Read the model definition and answer for the solid it produces. Units are mm, in the model's axes. Face numbers are marked on the shaded views. A direction names the side the tool comes from. Coordinates: 2 decimals unless noted, no trailing zeros. Order: outer loops, then holes, each group sorted by start corner. A loop starts at its lowest first (then second) coordinate and runs counter-clockwise, first axis right, second up. Notation, with made-up numbers: (79.5, 17) -> (121.5, 17) arc R15 ccw to (121.5, 30) -> close; hole circle Ø2 at (4, -16). An arc over 180 degrees is marked (long way). Answer in a Markdown table with one row per item.
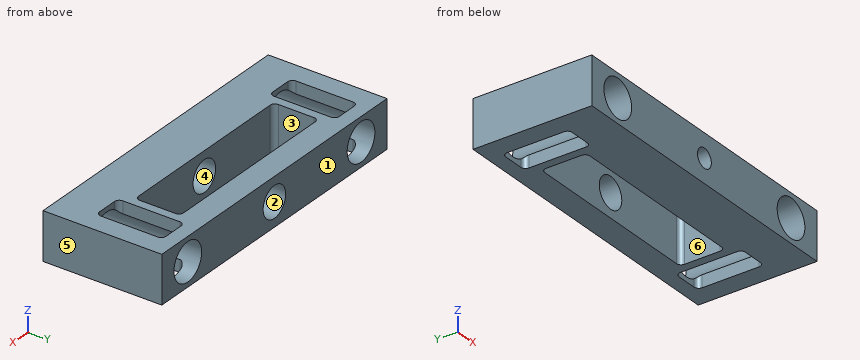
from build123d import *

# Parameters (mm, degrees)
SKETCH1_W                = 130
SKETCH1_H                = 50
BOSS_EXTRUDE1_DEPTH      = 10
BOSS_EXTRUDE1_DEPTH_BACK = 10
SKETCH2_R                = 8
CUT_EXTRUDE1_DEPTH       = 1
CUT_EXTRUDE1_DEPTH_BACK  = 51
CUT_EXTRUDE2_DEPTH       = 23
SKETCH5_R                = 4
CUT_EXTRUDE3_DEPTH       = 1.0000001
CUT_EXTRUDE3_DEPTH_BACK  = 51.0000001
SKETCH6_R                = 6.5
CUT_EXTRUDE4_DEPTH       = 37.5


with BuildPart() as part:
    # Sketch1 → Boss-Extrude1 (new body, two sides)
    with BuildSketch(Plane.XY) as boss_extrude1_sk:
        with Locations((0, -5)):
            Rectangle(SKETCH1_W, SKETCH1_H)
        with BuildLine():
            Line((38, 9.5), (-38, 9.5))
            ThreePointArc((-38, 9.5), (-39.414213562, 8.914213562), (-40, 7.5))
            Line((-40, 7.5), (-40, -7.5))
            ThreePointArc((-40, -7.5), (-39.414213562, -8.914213562), (-38, -9.5))
            Line((-38, -9.5), (38, -9.5))
            ThreePointArc((38, -9.5), (39.414213562, -8.914213562), (40, -7.5))
            Line((40, -7.5), (40, 7.5))
            ThreePointArc((40, 7.5), (39.414213562, 8.914213562), (38, 9.5))
        make_face(mode=Mode.SUBTRACT)
    extrude(amount=BOSS_EXTRUDE1_DEPTH)
    extrude(boss_extrude1_sk.sketch, amount=-BOSS_EXTRUDE1_DEPTH_BACK)

    # Sketch2 → Cut-Extrude1 (cut, two sides)
    with BuildSketch(Plane(origin=(0, 20, 0), x_dir=(1, 0, 0), z_dir=(0, 1, 0))) as cut_extrude1_sk:
        with Locations((-50, 0)):
            Circle(SKETCH2_R)
        with Locations((50, 0)):
            Circle(SKETCH2_R)
    extrude(amount=CUT_EXTRUDE1_DEPTH, mode=Mode.SUBTRACT)
    extrude(cut_extrude1_sk.sketch, amount=-CUT_EXTRUDE1_DEPTH_BACK, mode=Mode.SUBTRACT)

    # Sketch4 → Cut-Extrude2 (cut)
    with BuildSketch(Plane(origin=(0, 0, -10), x_dir=(-1, 0, 0), z_dir=(0, 0, -1))):
        with BuildLine():
            Line((-45.65, 14), (-54.35, 14))
            ThreePointArc((-54.35, 14), (-55.764213562, 13.414213562), (-56.35, 12))
            Line((-56.35, 12), (-56.35, -12))
            ThreePointArc((-56.35, -12), (-55.764213562, -13.414213562), (-54.35, -14))
            Line((-54.35, -14), (-45.65, -14))
            ThreePointArc((-45.65, -14), (-44.235786438, -13.414213562), (-43.65, -12))
            Line((-43.65, -12), (-43.65, 12))
            ThreePointArc((-43.65, 12), (-44.235786438, 13.414213562), (-45.65, 14))
        make_face()
        with BuildLine():
            Line((56.35, 12), (56.35, -12))
            ThreePointArc((56.35, -12), (55.764213562, -13.414213562), (54.35, -14))
            Line((54.35, -14), (45.65, -14))
            ThreePointArc((45.65, -14), (44.235786438, -13.414213562), (43.65, -12))
            Line((43.65, -12), (43.65, 12))
            ThreePointArc((43.65, 12), (44.235786438, 13.414213562), (45.65, 14))
            Line((45.65, 14), (54.35, 14))
            ThreePointArc((54.35, 14), (55.764213562, 13.414213562), (56.35, 12))
        make_face()
    extrude(amount=-CUT_EXTRUDE2_DEPTH, mode=Mode.SUBTRACT)

    # Sketch5 → Cut-Extrude3 (cut, two sides)
    with BuildSketch(Plane(origin=(0, 20, 0), x_dir=(1, 0, 0), z_dir=(0, 1, 0))) as cut_extrude3_sk:
        Circle(SKETCH5_R)
    extrude(amount=CUT_EXTRUDE3_DEPTH, mode=Mode.SUBTRACT)
    extrude(cut_extrude3_sk.sketch, amount=-CUT_EXTRUDE3_DEPTH_BACK, mode=Mode.SUBTRACT)

    # Sketch6 → Cut-Extrude4 (cut)
    with BuildSketch(Plane(origin=(0, 20, 0), x_dir=(1, 0, 0), z_dir=(0, 1, 0))):
        Circle(SKETCH6_R)
    extrude(amount=-CUT_EXTRUDE4_DEPTH, mode=Mode.SUBTRACT)


solid = part.part
Q1. For the marked faces 4, 5 and 6, determine the directions among +Z, -Z, +X, -X, +Y, -Y from which every point of the face is accessible in a straight line to the end or side of a thin tool.
Outcome:
| item | result |
|---|---|
| face 4 | +Y |
| face 5 | +Z, -Z, +X, +Y, -Y |
| face 6 | +Z, -Z |
Q2. Given pin 1 (1 mm diameter, centred on x = 4.5, z = -2, fed in from +Y), flat-ended and moving along its own axis, determine where the tip first touches the part or whether it passes through.
Outcome:
| item | result |
|---|---|
| pin 1 | y = -17.5 |
Q3. The part is cut by section B-B (y = -0.5). Write down the section's boundary in (x, z), then the cut area to 3 significant figures.
Outcome:
| item | result |
|---|---|
| outline | (-65, -10) -> (-56.35, -10) -> (-56.35, -4.87) arc R8 cw to (-56.35, 4.87) -> (-56.35, 10) -> (-65, 10) -> close; (-43.65, -10) -> (-40, -10) -> (-40, 10) -> (-43.65, 10) -> (-43.65, 4.87) arc R8 cw to (-43.65, -4.87) -> close; (40, -10) -> (43.65, -10) -> (43.65, -4.87) arc R8 cw to (43.65, 4.87) -> (43.65, 10) -> (40, 10) -> close; (56.35, -10) -> (65, -10) -> (65, 10) -> (56.35, 10) -> (56.35, 4.87) arc R8 cw to (56.35, -4.87) -> close |
| area | 448 mm² |
Q4. The part is cut by section A-A (z = 0). Give the number of separate pieces and of enclosed holes in the cut face, then the cut area to 3 significant figures.
Outcome:
| item | result |
|---|---|
| separate pieces | 4 |
| enclosed holes | 0 |
| area | 3,040 mm² |
Q5. For a pull along Y with two mould halves and no side action, classify the marked faces 1, 2 and 3 as pulls with the +Y half, pulls with the -Y half, needs draft (parallel to the pull), parting line crosses it, or undercut.
Outcome:
| item | result |
|---|---|
| face 1 | pulls with the +Y half |
| face 2 | needs draft |
| face 3 | undercut |
Q6. The part is cut by section C-C (x = -50). Write down the section's boundary in (y, z), then the cut area to 3 significant figures.
Outcome:
| item | result |
|---|---|
| outline | (-30, -10) -> (-14, -10) -> (-14, -8) -> (-30, -8) -> close; (-30, 8) -> (-14, 8) -> (-14, 10) -> (-30, 10) -> close; (14, -10) -> (20, -10) -> (20, -8) -> (14, -8) -> close; (14, 8) -> (20, 8) -> (20, 10) -> (14, 10) -> close |
| area | 88.0 mm² |
Q7. The part is cut by section D-D (y = -20). Write down the section's boundary in (x, z), then the cut area to 3 significant figures.
Outcome:
| item | result |
|---|---|
| outline | (-65, -10) -> (65, -10) -> (65, 10) -> (-65, 10) -> close; hole circle Ø16 at (-50, 0); hole circle Ø8 at (0, 0); hole circle Ø16 at (50, 0) |
| area | 2,150 mm² |
Q8. Consider line 1 (X direction, y = 3.5, z = 0); line 2 (X direction, y = -22, z = 0); line 3 (Z direction, x = 0, y = -15.25). Determine where each line is inside the solid, lowest interval first.
Outcome:
| item | result |
|---|---|
| line 1 | -65 to -58, -42 to -40, 40 to 42, 58 to 65 |
| line 2 | -65 to -58, -42 to -4, 4 to 42, 58 to 65 |
| line 3 | -10 to -6.5, 6.5 to 10 |
